Autodesk Inventor part; units mm, degrees
ref_plane "YZ Plane" through (0, 0, 0) normal (1, 0, 0) x (0, 1, 0)
ref_plane "XZ Plane" through (0, 0, 0) normal (0, 1, 0) x (-1, 0, 0)
ref_plane "XY Plane" through (0, 0, 0) normal (0, 0, 1) x (1, 0, 0)
sketch "Sketch1" plane through (0, 0, 0) normal (0, 1, 0) x (-1, 0, 0)
  line L0 (11.75, 16) -> (-11.75, 16)
  line L1 (-11.75, 16) -> (-11.75, -16)
  line L2 (-11.75, -16) -> (11.75, -16)
  line L3 (11.75, -16) -> (11.75, 16)
  point P0 (0, 0)
  dimension "d0" = 23.5
  dimension "d1" = 32
extrude "Extrusion1" add sketch "Sketch1" along normal blind 1.5
sketch "Sketch2" plane through (0, 1.5, 0) normal (0, 1, 0) x (1, 0, 0)
  line L0 (-11.5, 11.5) -> (11.5, 11.5)
  line L1 (11.5, 11.5) -> (11.5, -11.5)
  line L2 (11.5, -11.5) -> (-11.5, -11.5)
  line L3 (-11.5, -11.5) -> (-11.5, 11.5)
  line L4 (-11.5, 11.5) -> (11.5, -11.5) construction
  line L5 (11.5, 11.5) -> (-11.5, -11.5) construction
  point P0 (0, 0)
  dimension "d4" = 23
  dimension "d5" = 23
extrude "Extrusion2" add sketch "Sketch2" along normal blind 3.5
sketch "Sketch3" plane through (0, 5, 0) normal (0, 1, 0) x (1, 0, 0)
  circle A0 centre (0, 0) radius 11.5
  dimension "d8" = 23
extrude "Extrusion3" add sketch "Sketch3" along normal blind 12
fillet "Fillet1" radius 10 1 edges at (-11.5, 17, 0)
sketch "Sketch4" plane through (0, 0, 0) normal (0, -1, 0) x (1, 0, 0)
  line L0 (11.75, -16) -> (-11.75, -16)
  line L1 (-11.75, -16) -> (-11.75, 16)
  circle A0 centre (-11.75, -16) radius 2
  line L2 (-11.75, 16) -> (11.75, 16)
  circle A1 centre (-11.75, 16) radius 2
  circle A2 centre (11.75, 16) radius 2
  line L3 (11.75, -16) -> (4.75, -16)
  line L4 (4.75, -16) -> (4.75, -14)
  line L5 (4.75, -14) -> (11.75, -14)
  line L6 (11.75, -14) -> (11.75, -16)
  line L7 (11.75, 16) -> (11.75, -16)
  line L8 (4.75, -15.5) -> (3.0316, -15.5)
  point P0 (0, 0)
  dimension "d13" = 4
  dimension "d14" = 4
  dimension "d20" = 4
  dimension "d21" = 7
  dimension "d22" = 2
  dimension "d36" = 0.5
sketch "Sketch5" plane through (0, 0, 0) normal (0, -1, 0) x (1, 0, 0)
  line L0 (-9.743, 3.5) -> (-9.743, -3.5)
  line L1 (-9.743, -3.5) -> (-11.743, -3.5)
  line L2 (-11.743, -3.5) -> (-11.743, 3.5)
  line L3 (-11.743, 3.5) -> (-9.743, 3.5)
  line L4 (-11.75, -16) -> (-11.75, 16)
  point P0 (0, 0)
  point P1 (-11.75, 0)
  dimension "d16" = 7
  dimension "d17" = 2
extrude "Extrusion4" add sketch "Sketch5" along normal blind 2
extrude "Extrusion5" add sketch "Sketch4" along normal blind 2 contours L0 L4 L5 L6
sketch "Sketch6" plane through (0, 0, 0) normal (0, -1, 0) x (1, 0, 0)
  circle A0 centre (9.525, 12.7) radius 2
  circle A1 centre (-9.525, 12.7) radius 2
  circle A2 centre (-9.525, -12.7) radius 2
  point P0 (0, 0)
  dimension "d26" = 4
  dimension "d27" = 4
  dimension "d28" = 4
extrude "Extrusion6" add sketch "Sketch6" along normal blind 10
sketch "Sketch7" plane through (0, -2, 0) normal (0, -1, 0) x (1, 0, 0)
  circle A0 centre (-10.8242, 0) radius 0.25
  circle A1 centre (-10.8242, 2.1954) radius 0.25
  circle A2 centre (-10.8242, -1.9618) radius 0.25
  point P0 (0, 0)
  dimension "d31" = 0.5
  dimension "d32" = 0.5
  dimension "d33" = 0.5
extrude "Extrusion7" add sketch "Sketch7" along normal blind 8
sketch "Sketch8" plane through (0, 1.5, 0) normal (0, 1, 0) x (1, 0, 0)
  circle A0 centre (0, 14.5) radius 1
  line L0 (0, 11.5) -> (-11.5, 11.5)
  circle A1 centre (0, -14.5) radius 1
  line L1 (-11.5, -11.5) -> (0, -11.5)
  point P0 (0, 0)
  dimension "d37" = 2
  dimension "d38" = 2
hole "Hole1" at (0, 1.5, -14.5) at (0, 1.5, 14.5) direction (0, -1, 0) diameter 2 end through all
properties part number "MotionSensor"
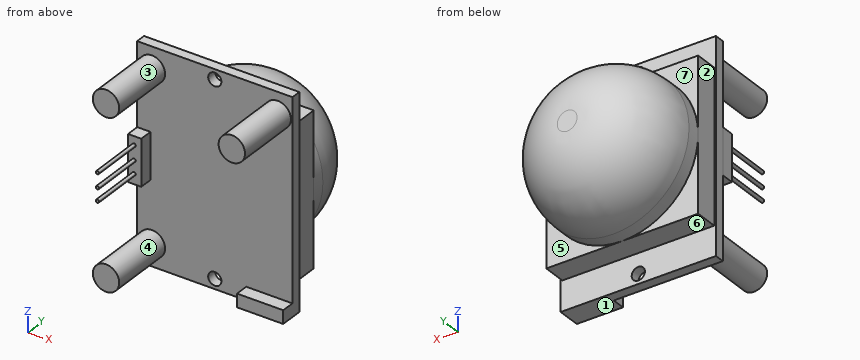
Part model, mm, in its own coordinate system. Face numbers are marked on the shaded views. A direction names the side the tool comes from. Coordinates: 2 decimals unless noted, no trailing zeros. Order: outer loops, then holes, each group sorted by start corner. A loop starts at its lowest first (then second) coordinate and runs counter-clockwise, first axis right, second up.
(1) Pull direction X, two halves, no side cores. Call the marked faces 1, 2 and 3: pulls with the +X half, pulls with the -X half, needs draft (parallel to the pull), parting line crosses it, or undercut.
Check sheet entries:
face 1: needs draft
face 2: pulls with the -X half
face 3: undercut
(2) Slice it at B-B, the plane y = -6. Write the cut outline in (x, z) (3 decimals), and give its area (3 significant figures).
Check sheet entries:
outline: circle Ø4 at (-9.525, -12.7); circle Ø4 at (-9.525, 12.7); circle Ø0.5 at (-10.824, -1.962); circle Ø0.5 at (-10.824, 0); circle Ø0.5 at (-10.824, 2.195); circle Ø4 at (9.525, 12.7)
area: 38.3 mm2
(3) Pin check, flat tips, straight feed: pin 1 Ø1 at (y, z) = (2.5, -4) entering from -X; pin 2 Ø2.5 at (x, z) = (0, -14.5) entering from -Y; pin 3 Ø1 at (y, z) = (-1, -0.5) entering from -X; pin 4 Ø10 at (y, z) = (-3.5, 0.5) entering from -X. Stop position of each tip, or through.
Check sheet entries:
pin 1: stops at x = -11.5
pin 2: stops at y = 0
pin 3: stops at x = -11.74
pin 4: stops at x = -11.75
(4) Slice it at A-A, the plane z = 12.7. Write the cut outline in (x, y) (3 decimals), and give its area (3 significant figures).
Check sheet entries:
outline: (-11.75, 0) - (-11.525, 0) - (-11.525, -10) - (-7.525, -10) - (-7.525, 0) - (7.525, 0) - (7.525, -10) - (11.525, -10) - (11.525, 0) - (11.75, 0) - (11.75, 1.5) - (-11.75, 1.5) - close
area: 115 mm2
(5) Probe L1, parallel to Z at x = 0, y = 0.95; L2, parallel to X at y = 0.5, z = -14.5; L3, parallel to Y at x = 5.5, z = -13. List the from-to ranges inside material, lowest first.
Check sheet entries:
L1: z = -16 to -15.5, -13.5 to 13.5, 15.5 to 16
L2: x = -11.75 to -1, 1 to 11.75
L3: y = 0 to 1.5
(6) Slice it at C-C, the plane z = -12.7. Write the cut outline in (x, y) (3 decimals).
Check sheet entries:
outline: (-11.75, 0) - (-11.525, 0) - (-11.525, -10) - (-7.525, -10) - (-7.525, 0) - (11.75, 0) - (11.75, 1.5) - (-11.75, 1.5) - close
(7) Tool access for the marked faces 4, 5, 6 and 7: list every direction of +Z, -Z, +X, -X, +Y, -Y with a clear straight run to the whole face (end or side of a thin tool).
Check sheet entries:
face 4: -Y
face 5: -Z, +X, +Y
face 6: -Z, +X, -X, +Y
face 7: +Z, -X, +Y
